from build123d import *

# Parameters (mm, degrees)
CROQUIS1_R              = 6
SALIENTE_EXTRUIR1_DEPTH = 6.5
CROQUIS2_R              = 9
SALIENTE_EXTRUIR2_DEPTH = 1.25
CROQUIS3_R              = 9
SALIENTE_EXTRUIR3_DEPTH = 1.25
CROQUIS4_R              = 2.5
CORTAR_EXTRUIR1_DEPTH   = 10


with BuildPart() as part:
    # Croquis1 → Saliente-Extruir1 (new body)
    with BuildSketch(Plane.XY):
        Circle(CROQUIS1_R)
    extrude(amount=SALIENTE_EXTRUIR1_DEPTH)

    # Croquis2 → Saliente-Extruir2 (add)
    with BuildSketch(Plane.XY.offset(6.5)):
        Circle(CROQUIS2_R)
    extrude(amount=SALIENTE_EXTRUIR2_DEPTH)

    # Croquis3 → Saliente-Extruir3 (add)
    with BuildSketch(Plane(origin=(0, 0, 0), x_dir=(-1, 0, 0), z_dir=(0, 0, -1))):
        Circle(CROQUIS3_R)
    extrude(amount=SALIENTE_EXTRUIR3_DEPTH)

    # Croquis4 → Cortar-Extruir1 (cut, through all)
    with BuildSketch(Plane(origin=(0, 0, -1.25), x_dir=(-1, 0, 0), z_dir=(0, 0, -1))):
        Circle(CROQUIS4_R)
    extrude(amount=-CORTAR_EXTRUIR1_DEPTH, mode=Mode.SUBTRACT)


solid = part.part
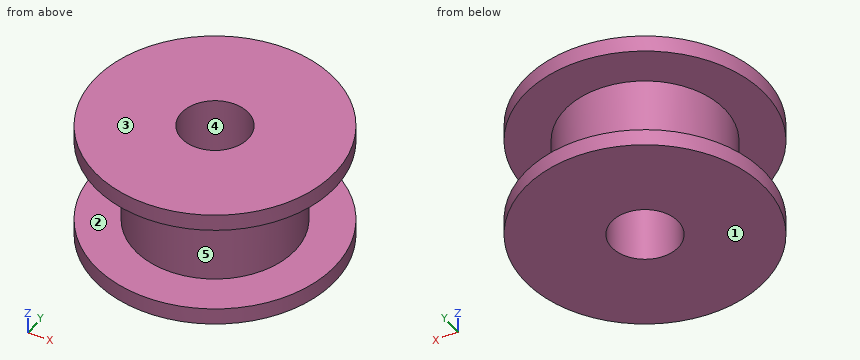
Geometry: final body of the model. Coordinates: model frame, mm. Face numbers are marked on the shaded views. A direction names the side the tool comes from. Give positions to 0.01 mm unless a question says otherwise; leave off trailing zeros. Loops run counter-clockwise (first coordinate to the right, second up) from the corner with the lowest first, then second, coordinate; pieces in that order, holes last. Notation, with made-up numbers: (-3.5, 38) - (37.5, 38) arc R13 ccw to (37.5, 51) - close; hole circle Ø1 at (-35.5, -29). An arc over 180 degrees is marked (long way). One line per question, with ' | ' between items. Start each with the question number.
(1) Reachability of the marked faces 4 and 5 from +Z, -Z, +X, -X, +Y, -Y: full face, straight path, thin tool, end or side. Return the list, or none.
(2) Pull-direction query (Z, two-part tool) for the marked faces 1, 2 and 3; classes: released by +Z, released by -Z, zero draft, split by the parting line, or undercut.
(3) Contact query for flat-ended pins moving along their axis: pin 1 (4 mm diameter, centred on x = 0, y = 0, fed in from -Z); pin 2 (1.5 mm diameter, centred on x = -6, z = 0.5, fed in from -Y); pin 3 (3 mm diameter, centred on y = 1, z = 3, fed in from -X). Output: stop coordinate, or through.
(4) Section query D-D on y = 5.25. Return loops of the section in (x, z).
(5) Section query A-A on y = 0. Return loops of the section in (x, z), then the cut area to 3 significant figures.
(6) Section query C-C on z = 0.5. Return loops of the section in (x, y).
(7) Ray query, line 1 (Y direction, x = 0, z = 4.25); line 2 (Z direction, x = -3.75, y = 5.5); line 3 (X direction, y = 0.75, z = 6). Return the intervals inside material, ascending. Write a range as from..to.
The answers:
1) face 4: +Z, -Z | face 5: none
2) face 1: released by -Z | face 2: undercut | face 3: released by +Z
3) pin 1: through | pin 2: y = -7.17 | pin 3: x = -6
4) outline: (-7.31, -1.25) - (7.31, -1.25) - (7.31, 0) - (2.9, 0) - (2.9, 6.5) - (7.31, 6.5) - (7.31, 7.75) - (-7.31, 7.75) - (-7.31, 6.5) - (-2.9, 6.5) - (-2.9, 0) - (-7.31, 0) - close
5) outline: (-9, -1.25) - (-2.5, -1.25) - (-2.5, 7.75) - (-9, 7.75) - (-9, 6.5) - (-6, 6.5) - (-6, 0) - (-9, 0) - close; (2.5, -1.25) - (9, -1.25) - (9, 0) - (6, 0) - (6, 6.5) - (9, 6.5) - (9, 7.75) - (2.5, 7.75) - close | area: 78.0 mm2
6) outline: circle Ø12 at (0, 0); hole circle Ø5 at (0, 0)
7) line 1: -6..-2.5, 2.5..6 | line 2: -1.25..0, 6.5..7.75 | line 3: -5.95..-2.38, 2.38..5.95
